The listing builds one solid part. Answer for the finished solid, in the listing's coordinates (mm). A direction names the side the tool comes from. Give positions to 0.01 mm unless a question says otherwise; leave off trailing zeros. Order: outer loops, then holes, each group sorted by start corner. A loop starts at its lowest first (then second) coordinate and runs counter-clockwise, first axis right, second up. Notation, with made-up numbers: (81, -6) -> (104, -6) arc R22 ccw to (104, 23) -> close; hole circle Ø1 at (29.5, -32). An arc over 180 degrees is marked (long way). Answer as a JSON object with one key per item and string values. Group by question number.
```python
from build123d import *

# Parameters (mm, degrees)
RESSALTO_EXTRUS_O1_DEPTH     = 5
RESSALTO_EXTRUS_O2_START     = -15
RESSALTO_EXTRUS_O2_OUTLINE_R = 1.9
RESSALTO_EXTRUS_O2_DEPTH     = 5
FILETE5_R                    = 1


# Read off the part's stored shape, not the designer's step: Ressalto-extrusão2
with BuildPart() as part:
    # Esboço1 → Ressalto-extrusão1 (new body)
    with BuildSketch(Plane.XY):
        with BuildLine():
            Line((4.587776734, -7.88962854), (4.587776734, -10))
            Line((4.587776734, -10), (-4.587776734, -10))
            Line((-4.587776734, -10), (-4.587776734, -7.88962854))
            ThreePointArc((-4.587776734, -7.88962854), (-9.126551039, 0), (-4.587776734, 7.88962854))
            Line((-4.587776734, 7.88962854), (-3.01610765, 5.186819319))
            ThreePointArc((-3.01610765, 5.186819319), (0, -6), (3.01610765, 5.186819319))
            Line((3.01610765, 5.186819319), (4.587776734, 7.88962854))
            ThreePointArc((4.587776734, 7.88962854), (9.126551039, 0), (4.587776734, -7.88962854))
        make_face()
    extrude(amount=RESSALTO_EXTRUS_O1_DEPTH)

    # Ressalto-extrusão2 outline → Ressalto-extrusão2 (add)
    with BuildSketch(Plane(origin=(0, 0, 0), x_dir=(1, 0, 0), z_dir=(0, 1, 0)).offset(RESSALTO_EXTRUS_O2_START)):
        with Locations((0, -2.5)):
            Circle(RESSALTO_EXTRUS_O2_OUTLINE_R)
    extrude(amount=RESSALTO_EXTRUS_O2_DEPTH)

    # Filete5
    filete5_edges = [part.edges().sort_by_distance(p)[0] for p in [
        (-1.9, -15, 2.5),
    ]]
    fillet(filete5_edges, radius=FILETE5_R)


solid = part.part
```
(1) For a pull along X with two mould halves and no side action, classify faces 1 (the cylindrical face through (9.126, 0.133, 2.465)), 2 (the flat face through (2, -10, 2)), 3 (the flat face through (-3.813, 6.557, 2.465)) as +X half, -X half, draft (parallel to the pull), parting line (faces both ways), or undercut.
(2) A cutting plane is placed at C-C (y = -12). Determine the outline of the cut face in (x, z).
(3) Find the intervals of material crossed by line 1 along Y through (x, z) = (4.75, 3.1); line 2 along Y through (x, z) = (-4.5, 2.6); line 3 along Y through (x, z) = (0, 2.95), in increasing order. Write a range as [from, to].
(4) A cutting plane is placed at B-B (z = 4.7). Determine the outline of the cut face in (x, y).
(5) Flat-ended cylindrical pins translate along their axes: pin 1 Ø1.7 at (y, z) = (-9, 3.5) entering from +X; pin 2 Ø3 at (y, z) = (-8.5, 1.5) entering from +X; pin 3 Ø1.1 at (y, z) = (-9, 2.5) entering from -X. Find the tip coordinate at first contact, or state that the pin passes through.
(6) A cutting plane is placed at A-A (y = 0). Determine the outline of the cut face in (x, z), and give its area (3 significant figures).
(7) A cutting plane is placed at D-D (x = -2.75). Determine the outline of the cut face in (y, z), and give its area (3 significant figures).
(8) Which of the six approach directions +Z, -Z, +X, -X, +Y, -Y give full straight-line access (tool end or side, diameter ignored) to faces 4 (the cylindrical face through (1.021, -12.028, 0.898)), 5 (the flat face through (4.588, -9, 2)), 6 (the flat face through (-4.588, -9, 2)), 7 (the flat face through (3.79, 6.52, 2.46))?
Check sheet entries:
{
 "1": {"face 1": "+X half", "face 2": "draft", "face 3": "undercut"},
 "2": {"outline": "circle Ø3.8 at (0, 2.5)"},
 "3": {"line 1": "y = [-7.79, -3.67], [3.67, 7.79]", "line 2": "y = [-10, -3.97], [3.97, 7.74]", "line 3": "y = [-15, -6]"},
 "4": {"outline": "(-4.59, -10) -> (4.59, -10) -> (4.59, -7.89) arc R9.13 ccw to (4.59, 7.89) -> (3.02, 5.19) arc R6 cw (long way) to (-3.02, 5.19) -> (-4.59, 7.89) arc R9.13 ccw to (-4.59, -7.89) -> close"},
 "5": {"pin 1": "stops at x = 4.59", "pin 2": "stops at x = 5.86", "pin 3": "stops at x = -4.59"},
 "6": {"outline": "(-9.13, 0) -> (-6, 0) -> (-6, 5) -> (-9.13, 5) -> close; (6, 0) -> (9.13, 0) -> (9.13, 5) -> (6, 5) -> close", "area": "31.3 mm2"},
 "7": {"outline": "(-10, 0) -> (-5.33, 0) -> (-5.33, 5) -> (-10, 5) -> close", "area": "23.3 mm2"},
 "8": {"face 4": "-Y", "face 5": "+Z, -Z, +X, -Y", "face 6": "+Z, -Z, -X, -Y", "face 7": "+Z, -Z, +Y"}
}
